For this review, use the dimensioned drawing (mm, ordinates from the lowest corner) and the shaded views. Give positions to 0.01 mm unless a question says otherwise; leave off trailing zeros. Write each loop counter-clockwise with the first axis right and the second up, starting at its lowest first coordinate (ties: lowest second). Pieces come first, ordered by that corner, then holes. Notation, with made-up numbers: (-8.5, 37) -> (49.5, 37) arc R20 cw to (49.5, 62) -> close; hole circle Ø10 at (5, -18.5). An arc over 180 degrees is marked (long way). Write each question's results on one line, items separated by ' | '. Start each with the question number.
(1) Take a section at C-C (z = 2.5). State the section outline as (x, y) points.
(2) Take a section at A-A (x = 6.35). State the section outline as (y, z) points.
(3) Clearance check with flat-ended pins moving along their axes: pin 1 (1 mm diameter, centred on x = 1.5, z = 4.5, fed in from +Y) (1 decimal); pin 2 (6.5 mm diameter, centred on x = 6.35, y = 6.35, fed in from +Z); pin 3 (3.5 mm diameter, centred on x = 6.35, y = 6.35, fed in from -Z); pin 4 (1 mm diameter, centred on x = 4, z = 5.5, fed in from +Y) (1 decimal). State where each tip first meets the part, or that it passes through.
(4) Mouldability with a two-part tool opening along Y and no side actions: class the marked faces 1, 2, 3 and 4 as released by +Y, released by -Y, zero draft, split by the parting line, or undercut.
(5) To check wall thickness, follow probe 1 along Y at (x, z) = (6.35, 1.9); probe 2 along Y at (x, z) = (4.5, 3.5) (1 decimal); probe 3 along Y at (x, z) = (1, 2.75). State the ranges of each line that lie inside material, in increasing order.
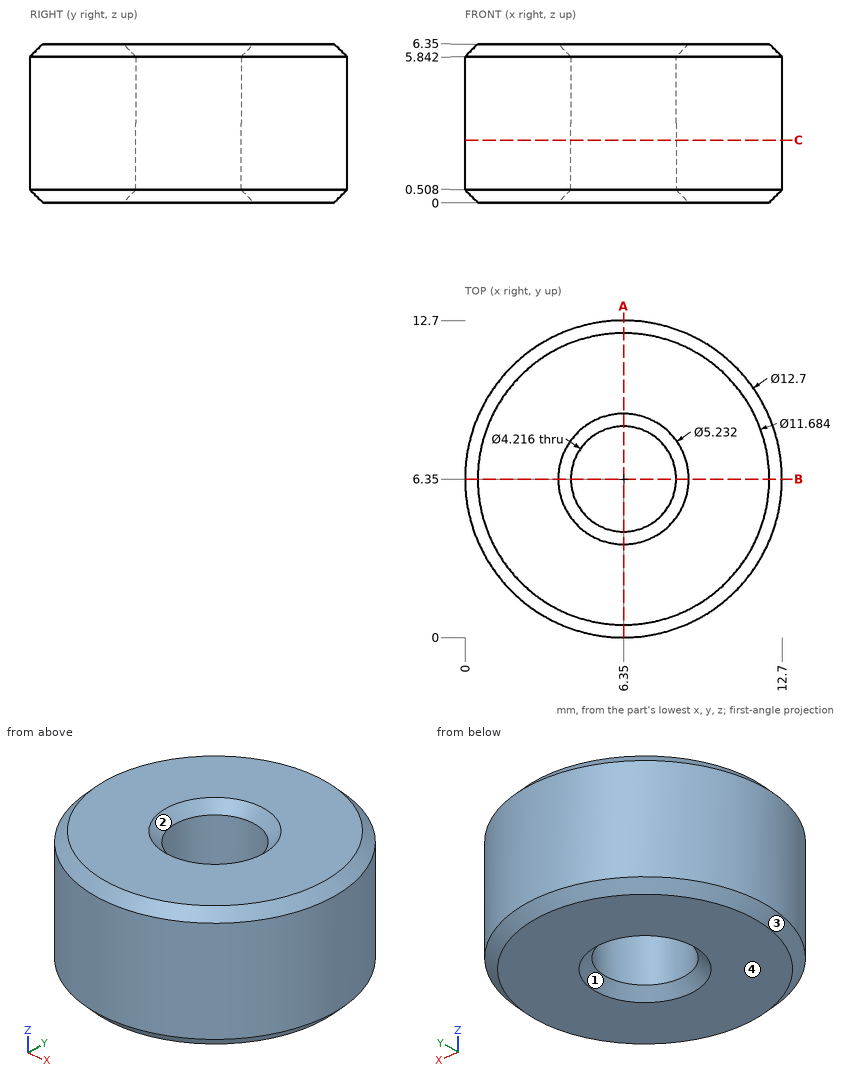
Report:
1) outline: circle Ø12.7 at (6.35, 6.35); hole circle Ø4.22 at (6.35, 6.35)
2) outline: (0, 0.51) -> (0.51, 0) -> (3.73, 0) -> (4.24, 0.51) -> (4.24, 5.84) -> (3.73, 6.35) -> (0.51, 6.35) -> (0, 5.84) -> close; (8.46, 0.51) -> (8.97, 0) -> (12.19, 0) -> (12.7, 0.51) -> (12.7, 5.84) -> (12.19, 6.35) -> (8.97, 6.35) -> (8.46, 5.84) -> close
3) pin 1: y = 11 | pin 2: z = 6.35 | pin 3: through | pin 4: y = 12.4
4) face 1: undercut | face 2: undercut | face 3: split by the parting line | face 4: zero draft
5) probe 1: 0 to 4.24, 8.46 to 12.7 | probe 2: 0.3 to 5.3, 7.4 to 12.4 | probe 3: 2.93 to 9.77
